Drawing for the job (mm, zero at the part's lowest x, y, z). Round coordinates to 2 decimals unless told otherwise and drop trailing zeros. Loops run counter-clockwise (first coordinate to the right, second up) from the corner with the lowest first, then second, coordinate; pieces in that order, holes last. Notation, with made-up numbers: M 8,29 L 38,29 A15 ccw 38,39 Z; hole C 31,82.5 d3. An arc over 180 degrees is marked long. Answer in a Markdown table with one row per item.
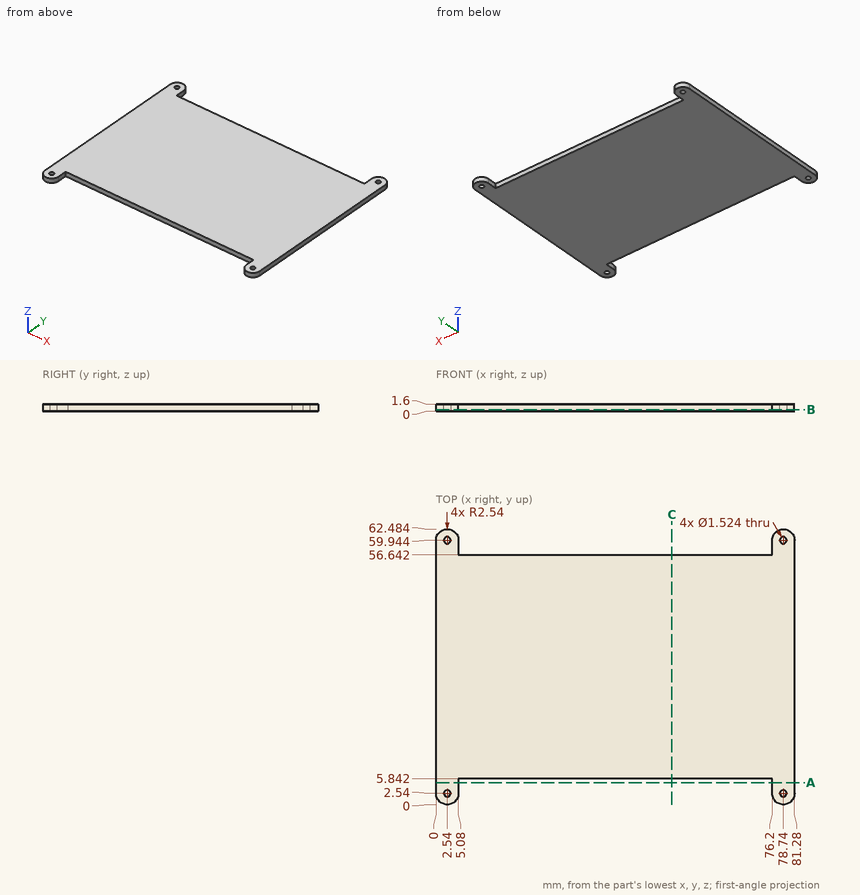
1. Saw through at B-B (z = 0.3). Write the cut outline in (x, y).
Verdict:
| item | result |
|---|---|
| outline | M 0,2.54 A2.54 ccw 5.08,2.54 L 5.08,5.84 L 76.2,5.84 L 76.2,2.54 A2.54 ccw 81.28,2.54 L 81.28,59.94 A2.54 ccw 76.2,59.94 L 76.2,56.64 L 5.08,56.64 L 5.08,59.94 A2.54 ccw 0,59.94 Z; hole C 2.54,2.54 d1.52; hole C 2.54,59.94 d1.52; hole C 78.74,2.54 d1.52; hole C 78.74,59.94 d1.52 |
2. Wall check: probe 1 along Y at (x, z) = (78.74, 0.75); probe 2 along Y at (x, z) = (42.5, 0.9). Give the ranges that are in metal, low to high.
Verdict:
| item | result |
|---|---|
| probe 1 | y = 0 to 1.78, 3.3 to 59.18, 60.71 to 62.48 |
| probe 2 | y = 5.84 to 56.64 |
3. Saw through at A-A (y = 5). Write the cut outline in (x, z), and give its area (3 significant figures).
Verdict:
| item | result |
|---|---|
| outline | M 0,0 L 5.08,0 L 5.08,1.6 L 0,1.6 Z; M 76.2,0 L 81.28,0 L 81.28,1.6 L 76.2,1.6 Z |
| area | 16.3 mm² |
4. Saw through at C-C (x = 53.5). Write the cut outline in (y, z).
Verdict:
| item | result |
|---|---|
| outline | M 5.84,0 L 56.64,0 L 56.64,1.6 L 5.84,1.6 Z |
5. Pin check, flat tip, straight feed: pin 1 (0.8 mm diameter, centred on x = 31, z = 1, fed in from -Y). Stop position of the tip, or through.
Verdict:
| item | result |
|---|---|
| pin 1 | stops at y = 5.84 |
